Autodesk Inventor part; units mm, degrees
ref_plane "YZ Plane" through (0, 0, 0) normal (1, 0, 0) x (0, 1, 0)
ref_plane "XZ Plane" through (0, 0, 0) normal (0, 1, 0) x (-1, 0, 0)
ref_plane "XY Plane" through (0, 0, 0) normal (0, 0, 1) x (1, 0, 0)
sketch "Sketch1" plane through (0, 0, 0) normal (0, 1, 0) x (-1, 0, 0)
  circle A0 centre (0, 0) radius 14.75
  line L0 (-20.25, 14.75) -> (-20.25, -14.75)
  line L1 (0, 14.75) -> (-20.25, 14.75)
  line L2 (0, -14.75) -> (-20.25, -14.75)
  point P0 (14.75, 0)
  dimension "d0" = 29.5
  dimension "d1" = 35
extrude "Extrusion1" add sketch "Sketch1" along normal blind 204.3
sketch "Sketch2" plane through (0, 0, 0) normal (0, -1, 0) x (1, 0, 0)
  line L0 (20.25, 20.275) -> (-36.05, 20.275)
  line L1 (-55.3, 6.365) -> (-55.3, 0) construction
  line L2 (-36.05, -20.275) -> (20.25, -20.275)
  line L3 (20.25, -20.275) -> (20.25, 20.275)
  line L4 (20.25, 14.75) -> (20.25, -14.75)
  line L5 (0, 0) -> (18.4964, 0) construction
  circle A0 centre (-36.05, 0) radius 19.25 construction
  arc A1 (-36.05, 20.275) -> (-36.05, -20.275) centre (-36.05, 0) ccw
  dimension "d6" = 38.5
  dimension "d4" = 40.55
  dimension "d5" = 75.55
extrude "Extrusion2" add sketch "Sketch2" along normal blind 22.3
sketch "Sketch3" plane through (0, 204.3, 0) normal (0, 1, 0) x (1, 0, 0)
  arc A0 (0, 14.75) -> (0, -14.75) centre (0, 0) ccw
  circle A1 centre (0, 0) radius 10.05
  dimension "d9" = 20.1
extrude "Extrusion3" cut sketch "Sketch3" against normal blind 150
sketch "Sketch4" plane through (0, 0, 0) normal (0, 1, 0) x (1, 0, 0)
  circle A0 centre (-36.05, 0) radius 19.05
  arc A1 (-36.05, 20.275) -> (-36.05, -20.275) centre (-36.05, 0) ccw
  point P0 (0, 0)
  dimension "d12" = 38.1
extrude "Extrusion4" add sketch "Sketch4" along normal blind 75.3
sketch "Sketch5" plane through (-36.05, 75.3, 0) normal (0, 1, 0) x (1, 0, 0)
  circle A0 centre (0, 0) radius 6.375
  circle A1 centre (0, 0) radius 19.05
  point P0 (36.05, 0)
  dimension "d15" = 12.75
extrude "Extrusion5" add sketch "Sketch5" along normal blind 2 contours A0
sketch "Sketch6" plane through (0, -22.3, 0) normal (0, -1, 0) x (1, 0, 0)
  circle A0 centre (0, 0) radius 10.05 construction
  line L0 (-8.9, -8.9) -> (8.9, -8.9)
  line L1 (8.9, -8.9) -> (8.9, 8.9)
  line L2 (8.9, 8.9) -> (-8.9, 8.9)
  line L3 (-8.9, 8.9) -> (-8.9, -8.9)
  line L4 (-8.9, -8.9) -> (8.9, 8.9) construction
  line L5 (8.9, -8.9) -> (-8.9, 8.9) construction
  arc A1 (-4.25, 8.9) -> (-8.9, 4.25) centre (-4.25, 4.25) ccw
  arc A2 (-8.9, -4.25) -> (-4.25, -8.9) centre (-4.25, -4.25) ccw
  arc A3 (4.25, -8.9) -> (8.9, -4.25) centre (4.25, -4.25) ccw
  arc A4 (8.9, 4.25) -> (4.25, 8.9) centre (4.25, 4.25) ccw
  point P0 (4.25, 8.9)
  point P1 (-4.25, -8.9)
  point P2 (8.9, -4.25)
  dimension "d18" = 17.8
  dimension "d19" = 17.8
  dimension "d22" = 360
  dimension "d24" = 8.5
extrude "Extrusion6" add sketch "Sketch6" along normal blind 18.8 contours A2 L3 A1 L2 A4 L1 A3 L0
fillet "Fillet1" radius 2 8 edges at (7.538, -22.3, 7.538) (8.9, -22.3, 0) (7.538, -22.3, -7.538) (0, -22.3, -8.9) (-7.538, -22.3, -7.538) (-8.9, -22.3, 0) (-7.538, -22.3, 7.538) (0, -22.3, 8.9)
sketch "Sketch7" plane through (-4.25, -41.1, 8.9) normal (0, 0, 1) x (1, 0, 0)
  circle A0 centre (4.25, 6.9) radius 3.175
  line L0 (8.5, 0) -> (0, 0)
  point P0 (4.25, 41.1)
  point P1 (4.25, 0)
  dimension "d28" = 6.9
  dimension "d29" = 6.35
extrude "Extrusion7" cut sketch "Sketch7" against normal through all
chamfer "Chamfer1" distance 1 angle 45 2 edges at (-3.175, -34.2, 8.9) (-3.175, -34.2, -8.9)
sketch "Sketch8" plane through (0, -22.3, 0) normal (0, -1, 0) x (1, 0, 0)
  line L0 (-50.7155, 14) -> (-50.7155, -14) construction
  arc A0 (-36.05, 20.275) -> (-36.05, -20.275) centre (-36.05, 0) ccw construction
  line L1 (-54.6626, 8.0403) -> (-46.7683, 17.2103)
  line L2 (-46.7683, 17.2103) -> (-59.6518, 28.3015)
  line L3 (-59.6518, 28.3015) -> (-67.5461, 19.1315)
  line L4 (-67.5461, 19.1315) -> (-54.6626, 8.0403)
  point P0 (0, 0)
  point P1 (-50.7155, 12.6253)
  dimension "d35" = 28
  dimension "d36" = 17
  dimension "d37" = 12.1
extrude "Extrusion8" add sketch "Sketch8" against normal up to surface (22.3 mm away)
properties part number "linear actuator"
Input: part model. Units: mm. Frame: model coordinates. A direction names the side the tool comes from. Coordinates: 2 decimals unless noted, no trailing zeros. Write each loop counter-clockwise with the first axis right and the second up, starting at its lowest first coordinate (ties: lowest second). Pieces come first, ordered by that corner, then holes.
1) Section D-D on x = -52. Output: boundary loops of the cut face in (y, z), and give its area (3 significant figures).
2) Pin query (flat end, axial travel): pin 1 Ø4 at (y, z) = (-30.5, -1.5) entering from -X; pin 2 Ø10 at (x, z) = (-3, 3.5) entering from +Y; pin 3 Ø5 at (x, z) = (-25.5, 3) entering from +Y. Return the tip coordinate at first contact, or that it passes through.
3) Set-up query: faces 5 (the flat face through (-17, 0, 4)), 6 (the flat face through (-8, -11, 20.275)), 7 (the flat face through (0, -29, 8.9)), 8 (the flat face through (-8.9, -33, 0)). Return all of +Z, -Z, +X, -X, +Y, -Y with unobstructed straight access to the full face (end or side cutting, diameter ignored); none if empty.
4) Mould query, pull axis X, two halves, no side actions, for faces 1 (the cylindrical face through (7.502, -32.582, 7.574)), 2 (the cylindrical face through (-51.17, 37.12, -11.59)), 3 (the flat face through (10, 101, -14.75)), 4 (the cylindrical face through (-7.502, -32.582, -7.574)). Classes: pulls with the +X half, pulls with the -X half, needs draft (parallel to the pull), parting line crosses it, or undercut.
5) Section C-C on y = 184.5. Output: boundary loops of the cut face in (x, z).
6) Section B-B on z = 0. Output: boundary loops of the cut face in (x, y) (3 decimals).
7) Material intervals for line 1 along X through (y, z) = (163, 0); line 2 along Z through (x, y) = (0, 161.5); line 3 along Y through (x, z) = (0, 3.75) (3 decimals), sorted ascending.
8) Section A-A on y = -34.2. Output: boundary loops of the cut face in (x, z) (3 decimals).
Check result:
1. outline: (-22.3, -12.52) - (0, -12.52) - (0, -10.42) - (75.3, -10.42) - (75.3, 10.42) - (0, 10.42) - (0, 21.71) - (-22.3, 21.71) - close
1. area: 2,330 mm2
2. pin 1: stops at x = -8.9
2. pin 2: stops at y = 54.3
2. pin 3: stops at y = 75.3
3. face 5: +Y
3. face 6: +Z, +X, +Y, -Y
3. face 7: +Z, +X, -X, -Y
3. face 8: +Z, -Z, -X, -Y
4. face 1: pulls with the +X half
4. face 2: undercut
4. face 3: needs draft
4. face 4: pulls with the -X half
5. outline: (0, -14.75) - (20.25, -14.75) - (20.25, 14.75) - (0, 14.75) arc R14.75 ccw to start; hole circle Ø20.1 at (0, 0)
6. outline: (-56.325, -22.3) - (-10.9, -22.3) arc R2 cw to (-8.9, -24.3) - (-8.9, -41.1) - (8.9, -41.1) - (8.9, -24.3) arc R2 cw to (10.9, -22.3) - (20.25, -22.3) - (20.25, 204.3) - (10.05, 204.3) - (10.05, 54.3) - (-10.05, 54.3) - (-10.05, 204.3) - (-14.75, 204.3) - (-14.75, 0) - (-17, 0) - (-17, 75.3) - (-29.675, 75.3) - (-29.675, 77.3) - (-42.425, 77.3) - (-42.425, 75.3) - (-55.1, 75.3) - (-55.1, 0) - (-56.325, 0) - close; hole circle Ø6.35 at (0, -34.2)
7. line 1: x = -14.75 to -10.05, 10.05 to 20.25
7. line 2: z = -14.75 to -10.05, 10.05 to 14.75
7. line 3: y = -41.1 to -37.375, -31.025 to 54.3
8. outline: (-8.9, -4.25) arc R4.65 ccw to (-4.25, -8.9) - (-4.175, -8.9) - (-3.175, -7.9) - (-3.175, 7.9) - (-4.175, 8.9) - (-4.25, 8.9) arc R4.65 ccw to (-8.9, 4.25) - close; (3.175, -7.9) - (4.175, -8.9) - (4.25, -8.9) arc R4.65 ccw to (8.9, -4.25) - (8.9, 4.25) arc R4.65 ccw to (4.25, 8.9) - (4.175, 8.9) - (3.175, 7.9) - close
